Geometry check sheet. Reference: the model listing, model coordinates, mm. A direction names the side the tool comes from. Round coordinates to 2 decimals unless told otherwise and drop trailing zeros. Order: outer loops, then holes, each group sorted by start corner. A loop starts at its lowest first (then second) coordinate and runs counter-clockwise, first axis right, second up.
```python
from build123d import *

# Parameters (mm, degrees)
F1_DEPTH = 95
F2_R     = 2.75
F2_R_2   = 10.5
F3_DEPTH = 6


with BuildPart() as f1:
    # F0 (on Front) → F1 (new body)
    with BuildSketch(Plane.XZ):
        Polygon((0, -6), (0, 0), (-90, 0), (-90, -25), (-81, -25), (-81, -6), align=None)
    extrude(amount=F1_DEPTH)

    # F2 (on face) → F3 (cut)
    with BuildSketch(Plane(origin=(0, 0, -6), x_dir=(1, 0, 0), z_dir=(0, 0, -1))):
        with Locations((-69, 72.5)):
            Circle(F2_R)
        with Locations((-38.5, 72.5)):
            Circle(F2_R)
        with Locations((-69, 22.5)):
            Circle(F2_R)
        with Locations((-38.5, 22.5)):
            Circle(F2_R)
        with Locations((-18.5, 47.5)):
            Circle(F2_R_2)
    extrude(amount=-F3_DEPTH, mode=Mode.SUBTRACT)


solid = f1.part
```
(1) Draft check along Y on faces 3 (the flat face through (-55, 0, -3)), 4 (the flat face through (-44, -47, 0)), 5 (the flat face through (-55, -95, -3)), 6 (the cylindrical face through (-13.655, -38.185, -3.042)). Enter one of: released by +Y, released by -Y, zero draft, split by the parting line, or undercut.
Returned:
face 3: released by +Y
face 4: zero draft
face 5: released by -Y
face 6: undercut
(2) Sectioned sample at D-D, the plane x = -9.5. Record the cut outline in (y, z), and give its area (3 significant figures).
Returned:
outline: (-95, -6) - (-52.91, -6) - (-52.91, 0) - (-95, 0) - close; (-42.09, -6) - (0, -6) - (0, 0) - (-42.09, 0) - close
area: 505 mm2
(3) Sectioned sample at A-A, the plane y = -47.5. Record the cut outline in (x, z), and give its area (3 significant figures).
Returned:
outline: (-90, -25) - (-81, -25) - (-81, -6) - (-29, -6) - (-29, 0) - (-90, 0) - close; (-8, -6) - (0, -6) - (0, 0) - (-8, 0) - close
area: 585 mm2
(4) Depth check by flat-ended pin: P1, Ø6.5, axis at x = -69, y = -22.5, coming from the -Z side; P2, Ø5.5, axis at y = -25, z = -13.5, coming from the +X side. Enter the tip coordinate at first touch or a pass-through.
Returned:
P1: stops at z = -6
P2: stops at x = -81
(5) Material ranges on line 1 (Y direction, x = -69, z = -2.4); line 2 (X direction, y = -47.5, z = -3.95); line 3 (X direction, y = -22, z = -5.25), recorded low to high.
Returned:
line 1: y = -95 to -75.25, -69.75 to -25.25, -19.75 to 0
line 2: x = -90 to -29, -8 to 0
line 3: x = -90 to -71.7, -66.3 to -41.2, -35.8 to 0
(6) Set-up check for faces 1 (the flat face through (-81, -47, -16)), 2 (the cylindrical face through (-41.247, -22.621, -3.042)): record each of +Z, -Z, +X, -X, +Y, -Y from which the full face is reachable in a straight line by a thin tool's end or side.
Returned:
face 1: -Z, +X, +Y, -Y
face 2: +Z, -Z
(7) Sectioned sample at B-B, the plane x = -69. Record the cut outline in (y, z).
Returned:
outline: (-95, -6) - (-75.25, -6) - (-75.25, 0) - (-95, 0) - close; (-69.75, -6) - (-25.25, -6) - (-25.25, 0) - (-69.75, 0) - close; (-19.75, -6) - (0, -6) - (0, 0) - (-19.75, 0) - close
(8) Sectioned sample at C-C, the plane z = -2.5. Record the cut outline in (x, y), and give its area (3 significant figures).
Returned:
outline: (-90, -95) - (0, -95) - (0, 0) - (-90, 0) - close; hole circle Ø5.5 at (-69, -72.5); hole circle Ø5.5 at (-69, -22.5); hole circle Ø5.5 at (-38.5, -72.5); hole circle Ø5.5 at (-38.5, -22.5); hole circle Ø21 at (-18.5, -47.5)
area: 8,110 mm2
